Geometry: see drawing. Coordinates: mm, zero at the bounding-box minimum. A direction names the side the tool comes from. Give positions to 0.01 mm unless a question says otherwise; leave off trailing zeros. Loops run counter-clockwise (first coordinate to the right, second up) from the corner with the lowest first, then second, coordinate; pieces in that order, holes last. Notation, with made-up numbers: M 40,72 L 60,72 A20 ccw 60,76 Z; hole C 22.5,7.25 d8. An arc over 180 degrees is marked long. Put each result on its own line as item: value.
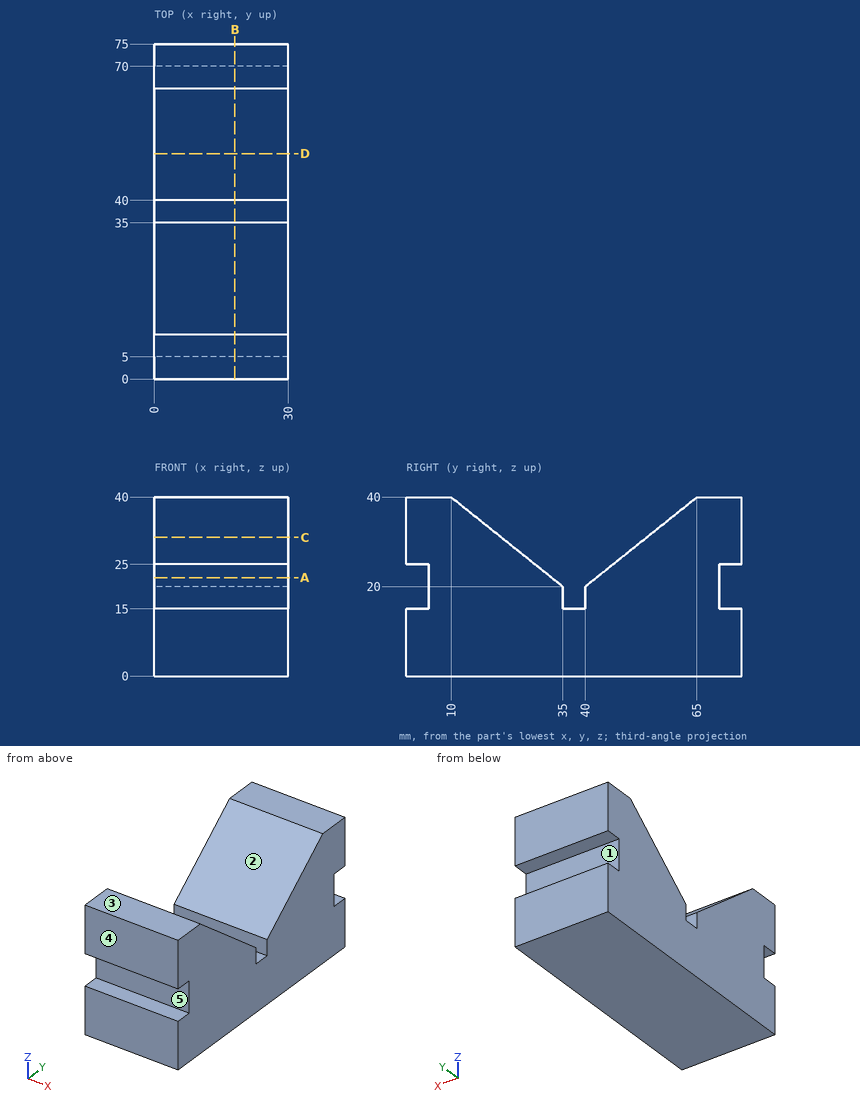
Item 1: Section C-C on z = 31. Output: boundary loops of the cut face in (x, y), then the cut area to 4 significant figures.
Output values:
outline: M 0,0 L 30,0 L 30,21.25 L 0,21.25 Z; M 0,53.75 L 30,53.75 L 30,75 L 0,75 Z
area: 1,275 mm²
Item 2: Line query: probe 1 along Y at (x, z) = (22, 16); probe 2 along Z at (x, y) = (28.25, 35.5); probe 3 along Y at (x, z) = (29.25, 38). Output: solid intervals per line, ascending. Write a range as [from, to].
Output values:
probe 1: [5, 35], [40, 70]
probe 2: [0, 15]
probe 3: [0, 12.5], [62.5, 75]
Item 3: Section A-A on z = 22. Output: boundary loops of the cut face in (x, y).
Output values:
outline: M 0,5 L 30,5 L 30,32.5 L 0,32.5 Z; M 0,42.5 L 30,42.5 L 30,70 L 0,70 Z
Item 4: Set-up query: the marked faces 4 and 5. Return all of +Z, -Z, +X, -X, +Y, -Y with unobstructed straight access to the full face (end or side cutting, diameter ignored); none if empty.
Output values:
face 4: +Z, -Z, +X, -X, -Y
face 5: +X, -X, -Y
Item 5: Pin query (flat end, axial travel): pin 1 Ø3 at (x, z) = (17, 19) entering from -Y. Return the tip coordinate at first contact, or that it passes through.
Output values:
pin 1: y = 5
Item 6: Section D-D on y = 50.5. Output: boundary loops of the cut face in (x, z), then the cut area to 3 significant figures.
Output values:
outline: M 0,0 L 30,0 L 30,28.4 L 0,28.4 Z
area: 852 mm²
Item 7: Section B-B on x = 18. Output: boundary loops of the cut face in (y, z).
Output values:
outline: M 0,0 L 75,0 L 75,15 L 70,15 L 70,25 L 75,25 L 75,40 L 65,40 L 40,20 L 40,15 L 35,15 L 35,20 L 10,40 L 0,40 L 0,25 L 5,25 L 5,15 L 0,15 Z
Item 8: Mould query, pull axis Y, two halves, no side actions, for the marked faces 1, 2 and 3. Classes: pulls with the +Y half, pulls with the -Y half, needs draft (parallel to the pull), parting line crosses it, or undercut.
Output values:
face 1: pulls with the +Y half
face 2: undercut
face 3: needs draft
